Geometry: final body of the model. Coordinates: model frame, mm. A direction names the side the tool comes from. Round coordinates to 2 decimals unless told otherwise and drop trailing zeros. Order: outer loops, then holes, each group sorted by start corner. A loop starts at its lowest first (then second) coordinate and runs counter-clockwise, first axis right, second up. Notation, with made-up numbers: M -25.75,-15.75 L -0.75,-15.75 A23 cw -0.75,-0.75 Z; hole C 69.5,68 d11. An arc over 180 degrees is marked long. Put each result on its own line as item: value. Start each with the question number.
1) Section A-A, the plane x = 9.5. Return loops of the section in (y, z).
2) Section C-C, the plane z = 259. Return loops of the section in (x, y), then the cut area to 3 significant figures.
3) Material intervals for probe 1 along Z at (x, y) = (128, -68); probe 2 along Y at (x, z) = (-9.5, 421.5); probe 3 along Z at (x, y) = (-422, 7), sorted ascending. Write a range as [from, to].
4) First-contact query: P1, Ø6, axis at x = 337, y = -22.5, coming from the -Z side; P2, Ø1.5, axis at x = 344.5, z = 378, coming from the -Y side; P3, Ø20.5, axis at y = -24.5, z = 8.5, coming from the -X side. Flat tips, straight axial feed; report the tip coordinate or a pass-through.
5) Access query for faces 1 (the flat face through (-8, -25.4, 338)), 2 (the flat face through (-421, 0, 25.4)), 3 (the flat face through (-4, 90, 25.4)), 4 (the flat face through (417, 0, 25.4)). Directions: +Z, -Z, +X, -X, +Y, -Y. A direction counts if a zero-diameter tool reaches every point of the face in a straight line with its end or side. Return the directions, or none.
6) Section B-B, the plane y = -53. Return loops of the section in (x, z).
from build123d import *

# Parameters (mm, degrees)
F0_W     = 584.2
F0_H     = 304.8
F1_DEPTH = 25.4
F2_W     = 254
F2_H     = 50.8
F2_W_2   = 584.2
F3_DEPTH = 635


with BuildPart() as f1:
    # F0 (on Top) → F1 (new body)
    with BuildSketch(Plane.XY):
        Rectangle(F0_W, F0_H)
    extrude(amount=F1_DEPTH)

    # F2 (on face) → F3 (join)
    with BuildSketch(Plane.XY.offset(25.4)):
        with Locations((-419.1, 0)):
            Rectangle(F2_W, F2_H)
        Rectangle(F2_W_2, F2_H)
        with Locations((419.1, 0)):
            Rectangle(F2_W, F2_H)
    extrude(amount=F3_DEPTH)


solid = f1.part
Result sheet:
1. outline: M -152.4,0 L 152.4,0 L 152.4,25.4 L 25.4,25.4 L 25.4,660.4 L -25.4,660.4 L -25.4,25.4 L -152.4,25.4 Z
2. outline: M -546.1,-25.4 L 546.1,-25.4 L 546.1,25.4 L -546.1,25.4 Z
2. area: 55,500 mm2
3. probe 1: z = [0, 25.4]
3. probe 2: y = [-25.4, 25.4]
3. probe 3: z = [25.4, 660.4]
4. P1: stops at z = 25.4
4. P2: stops at y = -25.4
4. P3: stops at x = -292.1
5. face 1: +Z, +X, -X, -Y
5. face 2: -Z, -X, +Y, -Y
5. face 3: +Z, +X, -X, +Y
5. face 4: -Z, +X, +Y, -Y
6. outline: M -292.1,0 L 292.1,0 L 292.1,25.4 L -292.1,25.4 Z
